from build123d import *

# Parameters (mm, degrees)
SKETCH001_W     = 45
SKETCH001_H     = 42
PAD001_DEPTH    = 26
SKETCH_W        = 45
SKETCH_H        = 45
PAD_DEPTH       = 26
SKETCH002_R     = 1
POCKET_DEPTH    = 26.001
POCKET001_DEPTH = 5


with BuildPart() as obj1:
    # Sketch001 → Pad001 (new body)
    with BuildSketch(Plane.XY):
        with Locations((22.5, 21)):
            Rectangle(SKETCH001_W, SKETCH001_H)
    extrude(amount=PAD001_DEPTH)


with BuildPart() as obj1_1:
    # Body001 placement: moved
    add(obj1.part.moved(Location((0, 3, -3))))


with BuildPart() as obj2:
    # Sketch → Pad (new body)
    with BuildSketch(Plane.XY):
        with Locations((22.5, 22.5)):
            Rectangle(SKETCH_W, SKETCH_H)
    extrude(amount=PAD_DEPTH)

    # Sketch002 → Pocket (cut, through all)
    with BuildSketch(Plane.XY.offset(26)):
        with Locations((22.5, 35)):
            Circle(SKETCH002_R)
    extrude(amount=-POCKET_DEPTH, mode=Mode.SUBTRACT)

    # Boolean: cut obj1
    add(obj1_1.part, mode=Mode.SUBTRACT)

    # Sketch003 (on Face4 of Boolean) → Pocket001 (cut)
    with BuildSketch(Plane.XY.offset(26)):
        Polygon((20.5, 45), (22.5, 42), (24.5, 45), align=None)
    extrude(amount=-POCKET001_DEPTH, mode=Mode.SUBTRACT)


solid = obj2.part
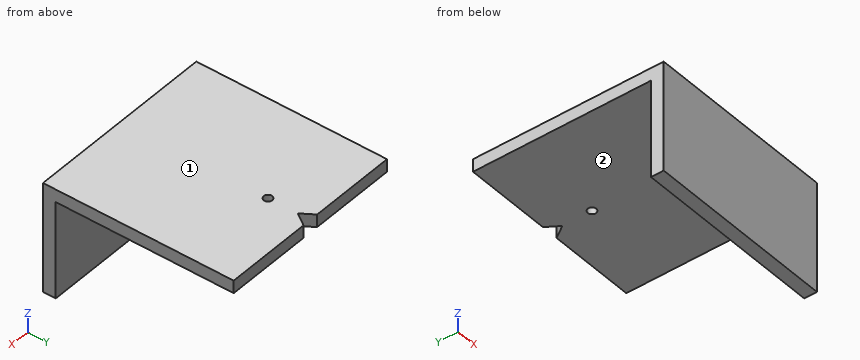
Check sheet for the modelled part. Datum: model origin and axes. Units: mm. Face numbers are marked on the shaded views. A direction names the side the tool comes from. Coordinates: 2 decimals unless noted, no trailing zeros. Write each loop counter-clockwise with the first axis right and the second up, starting at its lowest first coordinate (ties: lowest second). Pieces come first, ordered by that corner, then holes.
Item 1: Scan lines: probe 1 along Y at (x, z) = (37, 8); probe 2 along Z at (x, y) = (27, 22.5). Record each from-to range of solid material in increasing order.
Numbers:
probe 1: y = 0 to 3
probe 2: z = 23 to 26
Item 2: Cross-section at B-B on x = 17. Record the boundary of the cut face in (y, z).
Numbers:
outline: (0, 0) - (3, 0) - (3, 23) - (45, 23) - (45, 26) - (0, 26) - close
Item 3: Cross-section at A-A on y = 35. Record the boundary of the cut face in (x, z), then the cut area to 3 significant figures.
Numbers:
outline: (0, 23) - (21.5, 23) - (21.5, 26) - (0, 26) - close; (23.5, 23) - (45, 23) - (45, 26) - (23.5, 26) - close
area: 129 mm2
Item 4: Cross-section at D-D on y = 10. Record the boundary of the cut face in (x, z), then the cut area to 3 significant figures.
Numbers:
outline: (0, 23) - (45, 23) - (45, 26) - (0, 26) - close
area: 135 mm2
Item 5: Cross-section at C-C on z = 2. Record the boundary of the cut face in (x, y).
Numbers:
outline: (0, 0) - (45, 0) - (45, 3) - (0, 3) - close
Item 6: Depth check by flat-ended pin: pin 1 Ø1 at (x, y) = (17.5, 34) entering from -Z; pin 2 Ø1.5 at (x, z) = (19, 3) entering from +Y. Enter the tip coordinate at first touch or a pass-through.
Numbers:
pin 1: stops at z = 23
pin 2: stops at y = 3
Item 7: Access from +Z, -Z, +X, -X, +Y, -Y to the whole of each face (thin tool, end or side, straight path). Record for the marked faces 1 and 2.
Numbers:
face 1: +Z, +X, -X, +Y, -Y
face 2: -Z, +X, -X, +Y
